Check sheet for the drawn part. Datum: minimum x, y, z corner. Units: mm. A direction names the side the tool comes from. Coordinates: 2 decimals unless noted, no trailing zeros. Write each loop counter-clockwise with the first axis right and the second up, starting at its lowest first coordinate (ties: lowest second). Pieces come first, ordered by that corner, then holes. Notation, with made-up numbers: (-14.75, 81) - (21.25, 81) arc R20 cw to (21.25, 112) - close; hole circle Ø1 at (24, -9). An arc over 180 degrees is marked (long way). Use one line per item in the form item = value. Start each with the question number.
1. Go/stop test with flat-tipped pins: pin 1 Ø8 at (y, z) = (4, 7) entering from +X; pin 2 Ø3 at (x, z) = (7.5, 13.5) entering from +Y; pin 3 Ø6 at (x, y) = (5.5, 6.5) entering from +Z. Record where each tip stops, or that it passes through.
2. Cross-section at C-C on z = 10. Record the boundary of the cut face in (x, y).
3. Cross-section at D-D on z = 14.5. Record the boundary of the cut face in (x, y).
4. Scan lines: line 1 along Y through (x, z) = (1.55, 4); line 2 along X through (y, z) = (24.5, 16.5); line 3 along Y through (x, z) = (33, 9). Record each from-to range of solid material in increasing order.
5. Cross-section at A-A on y = 4. Record the boundary of the cut face in (x, z).
6. Cross-section at B-B on y = 23. Record the boundary of the cut face in (x, z), then the cut area to 3 significant figures.
7. Tool access check on the marked faces 1, 2 and 3. Record the directions out of +Z, -Z, +X, -X, +Y, -Y that give a thin tool (end or side, any length) a straight path to the whole face; none if there is none.
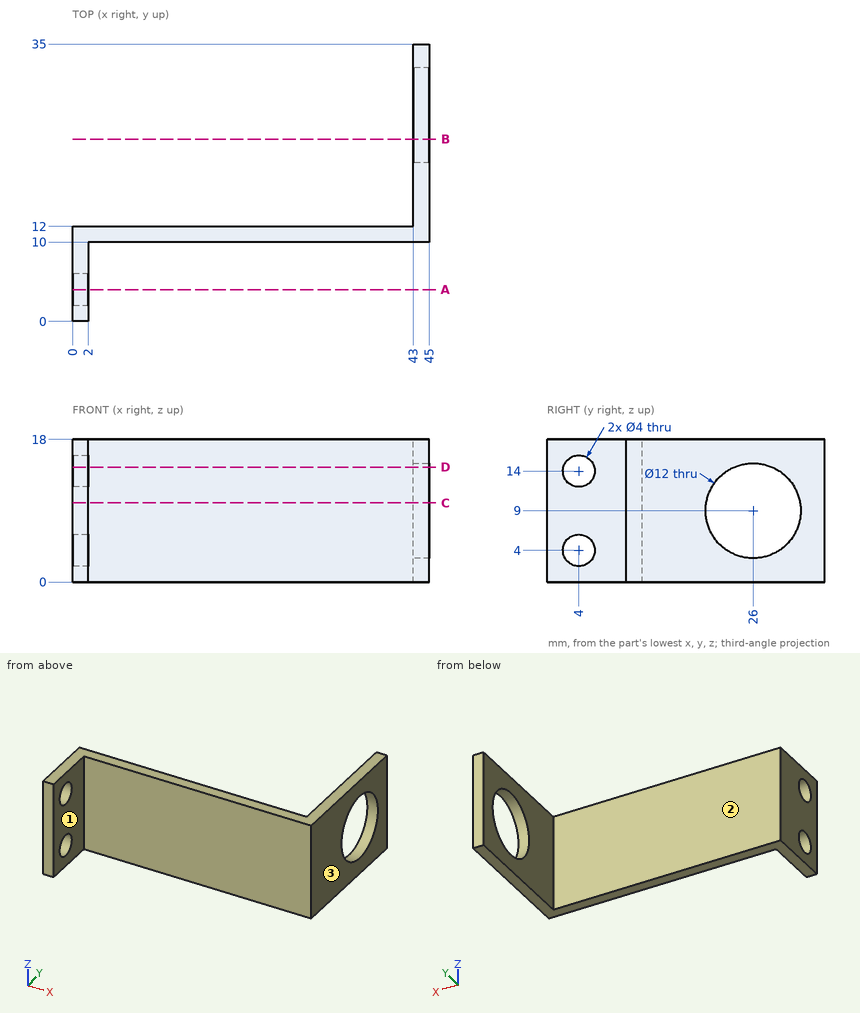
Final values:
q1.pin_1 = 2
q1.pin_2 = 12
q1.pin_3 = through
q2.outline = (0, 0) - (2, 0) - (2, 10) - (45, 10) - (45, 20.08) - (43, 20.08) - (43, 12) - (0, 12) - close; (43, 31.92) - (45, 31.92) - (45, 35) - (43, 35) - close
q3.outline = (0, 0) - (2, 0) - (2, 2.06) - (0, 2.06) - close; (0, 5.94) - (2, 5.94) - (2, 10) - (45, 10) - (45, 23.6) - (43, 23.6) - (43, 12) - (0, 12) - close; (43, 28.4) - (45, 28.4) - (45, 35) - (43, 35) - close
q4.line_1 = 0 to 2, 6 to 12
q4.line_2 = 43 to 45
q4.line_3 = 10 to 12
q5.outline = (0, 0) - (2, 0) - (2, 2) - (0, 2) - close; (0, 6) - (2, 6) - (2, 12) - (0, 12) - close; (0, 16) - (2, 16) - (2, 18) - (0, 18) - close
q6.outline = (43, 0) - (45, 0) - (45, 3.8) - (43, 3.8) - close; (43, 14.2) - (45, 14.2) - (45, 18) - (43, 18) - close
q6.area = 15.2 mm²
q7.face_1 = +Z, -Z, +X, -Y
q7.face_2 = +Z, -Z, -X, +Y
q7.face_3 = +Z, -Z, +X, +Y, -Y
